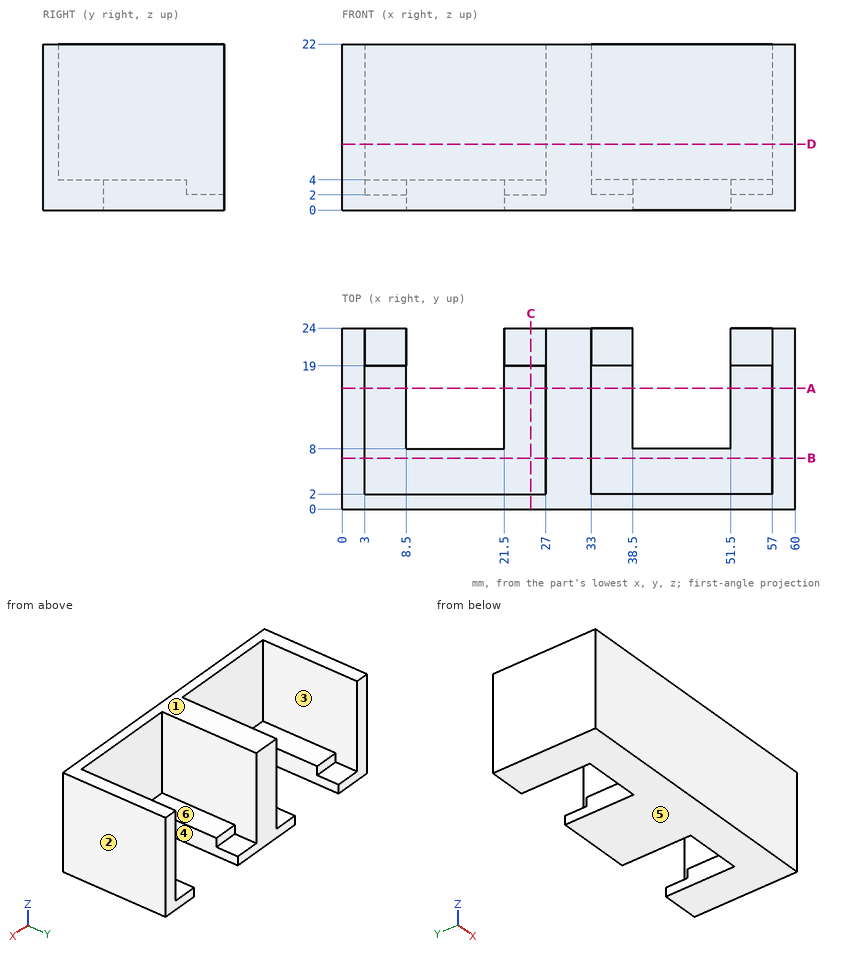
Source: three-view drawing plus pictorial views. Frame: mm from the lowest corner of the part. A direction names the side the tool comes from. Round coordinates to 2 decimals unless told otherwise and drop trailing zeros. Loops run counter-clockwise (first coordinate to the right, second up) from the corner with the lowest first, then second, coordinate; pieces in that order, holes last.
1. Section query D-D on z = 8.75. Output: boundary loops of the cut face in (x, y).
2. Ray query, L1, parallel to X at y = 11.75, z = 5; L2, parallel to X at y = 16.5, z = 3; L3, parallel to Y at x = 15.5, z = 4.25. Return the intervals inside material, ascending.
3. Mould query, pull axis X, two halves, no side actions, for the marked faces 1, 2 and 3. Classes: released by +X, released by -X, zero draft, split by the parting line, or undercut.
4. Section query C-C on x = 25. Output: boundary loops of the cut face in (y, z), and give its area (3 significant figures).
5. Section query B-B on y = 6.75. Output: boundary loops of the cut face in (x, z).
6. Access query for the marked faces 4, 5 and 6. Directions: +Z, -Z, +X, -X, +Y, -Y. A direction counts if a zero-diameter tool reaches every point of the face in a straight line with its end or side. Return the directions, or none.
7. Contact query for flat-ended pins moving along their axis: pin 1 (13.5 mm diameter, centred on x = 48, y = 12.5, fed in from +Z); pin 2 (4 mm diameter, centred on x = 44, z = 12.5, fed in from -Y); pin 3 (5.5 mm diameter, centred on x = 15.5, z = 16, fed in from +Y); pin 4 (1 mm diameter, centred on x = 53, z = 3, fed in from +Y). Output: stop coordinate, or through.
8. Section query A-A on y = 16. Output: boundary loops of the cut face in (x, z), and give its area (3 significant figures).
Answers below:
1. outline: (0, 0) - (60, 0) - (60, 24) - (57, 24) - (57, 2) - (33, 2) - (33, 24) - (27, 24) - (27, 2) - (3, 2) - (3, 24) - (0, 24) - close
2. L1: x = 0 to 3, 27 to 33, 57 to 60
2. L2: x = 0 to 8.5, 21.5 to 38.5, 51.5 to 60
2. L3: y = 0 to 2
3. face 1: zero draft
3. face 2: released by +X
3. face 3: undercut
4. outline: (0, 0) - (24, 0) - (24, 2) - (19, 2) - (19, 4) - (2, 4) - (2, 22) - (0, 22) - close
4. area: 122 mm2
5. outline: (0, 0) - (60, 0) - (60, 22) - (57, 22) - (57, 4) - (33, 4) - (33, 22) - (27, 22) - (27, 4) - (3, 4) - (3, 22) - (0, 22) - close
6. face 4: +Z, -Z, +Y
6. face 5: -Z, +X, -X, +Y, -Y
6. face 6: +Z, +Y
7. pin 1: stops at z = 4
7. pin 2: stops at y = 0
7. pin 3: stops at y = 2
7. pin 4: stops at y = 19
8. outline: (0, 0) - (8.5, 0) - (8.5, 4) - (3, 4) - (3, 22) - (0, 22) - close; (21.5, 0) - (38.5, 0) - (38.5, 4) - (33, 4) - (33, 22) - (27, 22) - (27, 4) - (21.5, 4) - close; (51.5, 0) - (60, 0) - (60, 22) - (57, 22) - (57, 4) - (51.5, 4) - close
8. area: 352 mm2
